Here's how the part is built. I have some questions about the finished solid (model axes, mm). Face numbers are marked on the shaded views. A direction names the side the tool comes from. Give positions to 0.01 mm unless a question says otherwise; leave off trailing zeros. Write each loop counter-clockwise with the first axis right and the second up, starting at its lowest first coordinate (ties: lowest second). Pieces come first, ordered by that corner, then holes. Notation, with made-up numbers: (43.25, 48) - (85.25, 48) arc R21 ccw to (85.25, 80) - close; hole circle Ø4 at (73, -17.5). An arc over 180 degrees is marked (long way). Write each question's results on one line, items separated by ' | '. Start each with the question number.
Item 1: We'd pull the mould along Y, two halves only. Please class the marked faces 4, 5 and 6: +Y half, -Y half, draft (parallel to the pull), parting line (faces both ways), or undercut.
Item 2: Which directions (+Z, -Z, +X, -X, +Y, -Y) give clear straight access to the entire face, cutting with the end or side of a thin tool? Please do the marked faces 1, 2 and 3.
Item 3: Please list where these lines run through material, in increasing order: line 1 along Y through (x, z) = (11.5, 1.15); line 2 along Z through (x, y) = (-6.5, 1.5).
Item 4: Suppose I cut it at D-D on y = 3.75. List the corners of the cut face in (x, z) for me, then the cut area to 3 significant figures.
Item 5: Suppose I cut it at A-A on x = 10.5. List the corners of the cut face in (y, z) for me, then the cut area to 3 significant figures.
Item 6: Will these pins go through, and if not, where does the flat tip stop? P1, Ø12.5, axis at x = -6, y = 3, coming from the +Z side; P2, Ø2, axis at x = -4, y = 4.5, coming from the +Z side.
Item 7: Suppose I cut it at C-C on z = 1.15. Count the separate pieces of the cut face and the enclosed holes in it, then the cut area to 3 significant figures.
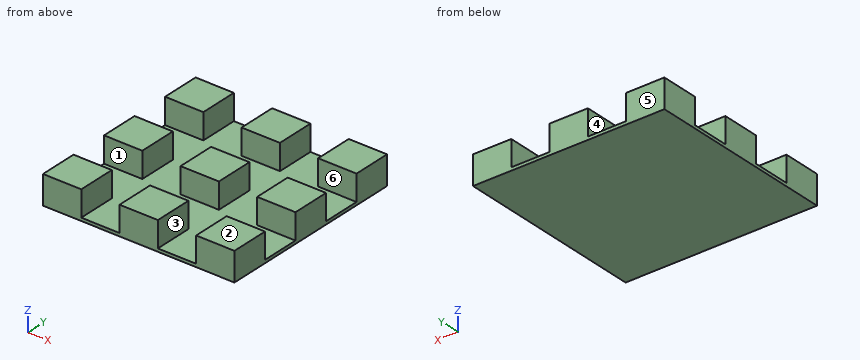
```python
from build123d import *

# Parameters (mm, degrees)
F0_W     = 5.08
F0_H     = 5.08
F1_DEPTH = 0.4064
F2_DEPTH = 3.81


with BuildPart() as f1:
    # F0 (on Top) → F1 (new body)
    with BuildSketch(Plane.XY):
        Polygon((-2.54, 12.7), (-7.62, 12.7), (-7.62, 7.62), (-12.7, 7.62), (-12.7, 2.54), (-7.62, 2.54), (-7.62, -2.54), (-12.7, -2.54), (-12.7, -7.62), (-7.62, -7.62), (-7.62, -12.7), (-2.54, -12.7), (-2.54, -7.62), (2.54, -7.62), (2.54, -12.7), (7.62, -12.7), (7.62, -7.62), (12.7, -7.62), (12.7, -2.54), (7.62, -2.54), (7.62, 2.54), (12.7, 2.54), (12.7, 7.62), (7.62, 7.62), (7.62, 12.7), (2.54, 12.7), (2.54, 7.62), (-2.54, 7.62), align=None)
        Rectangle(F0_W, F0_H, mode=Mode.SUBTRACT)
    extrude(amount=F1_DEPTH)

    # F0 (on Top) → F2 (join)
    with BuildSketch(Plane.XY):
        with Locations((-10.16, -10.16)):
            Rectangle(F0_W, F0_H)
        with Locations((-10.16, 0)):
            Rectangle(F0_W, F0_H)
        with Locations((-10.16, 10.16)):
            Rectangle(F0_W, F0_H)
        with Locations((0, 10.16)):
            Rectangle(F0_W, F0_H)
        Rectangle(F0_W, F0_H)
        with Locations((10.16, 0)):
            Rectangle(F0_W, F0_H)
        with Locations((10.16, 10.16)):
            Rectangle(F0_W, F0_H)
        with Locations((10.16, -10.16)):
            Rectangle(F0_W, F0_H)
        with Locations((0, -10.16)):
            Rectangle(F0_W, F0_H)
    extrude(amount=F2_DEPTH)


solid = f1.part
```
Checked values:
1) face 4: draft | face 5: +Y half | face 6: undercut
2) face 1: +Z, +X, -X | face 2: +Z, +X, -X, +Y, -Y | face 3: +Z, +Y, -Y
3) line 1: y = -12.7 to -7.62, -2.54 to 2.54, 7.62 to 12.7 | line 2: z = 0 to 0.41
4) outline: (-12.7, 0) - (12.7, 0) - (12.7, 0.41) - (-12.7, 0.41) - close | area: 10.3 mm^2
5) outline: (-12.7, 0) - (12.7, 0) - (12.7, 3.81) - (7.62, 3.81) - (7.62, 0.41) - (2.54, 0.41) - (2.54, 3.81) - (-2.54, 3.81) - (-2.54, 0.41) - (-7.62, 0.41) - (-7.62, 3.81) - (-12.7, 3.81) - close | area: 62.2 mm^2
6) P1: stops at z = 3.81 | P2: stops at z = 0.41
7) separate pieces: 9 | enclosed holes: 0 | area: 232 mm^2
